```python
from build123d import *

# Parameters (mm, degrees)
EXTRUDE_1_DEPTH               = 3
HOLE_WIZARD_M2_1_AT_2_COUNT   = 2
HOLE_WIZARD_M2_1_AT_2_PITCH   = 21
PATTERN_LINEAR_1_COUNT        = 3
PATTERN_LINEAR_1_PITCH        = 33
PATTERN_LINEAR_2_COUNT        = 3
PATTERN_LINEAR_2_PITCH        = 10.5
PATTERN_LINEAR_3_COUNT        = 2
PATTERN_LINEAR_3_PITCH        = 31.5
HOLE_WIZARD_M2_1_2_AT_2_COUNT = 2
HOLE_WIZARD_M2_1_2_AT_2_PITCH = 16.970562748
SKETCH_8_R                    = 17
CUT_EXTRUDE_1_DEPTH           = 1
SKETCH_9_R                    = 2.025
CUT_EXTRUDE_2_DEPTH           = 75.994999833
PATTERN_CIRCULAR_1_COUNT      = 2
PATTERN_CIRCULAR_1_ANGLE      = 90
FILLET_1_R                    = 4
CHAMFER_1_SIZE                = 1
SKETCH_11_W                   = 95
SKETCH_11_H                   = 18
CUT_EXTRUDE_3_DEPTH           = 76.028327984


with BuildPart() as part:
    # ｽｹｯﾁ1 → ﾎﾞｽ - 押し出し1 (new body)
    with BuildSketch(Plane(origin=(0, 0, 0), x_dir=(1, 0, 0), z_dir=(0, 1, 0))):
        with BuildLine():
            Line((-10.05, 0), (-39, 0))
            Line((-39, 0), (-47.5, 8.5))
            Line((-47.5, 8.5), (-47.5, 58))
            Line((-47.5, 58), (47.5, 58))
            Line((47.5, 58), (47.5, 8.5))
            Line((47.5, 8.5), (39, 0))
            Line((39, 0), (10.05, 0))
            ThreePointArc((10.05, 0), (0, 10.05), (-10.05, 0))
        make_face()
    extrude(amount=EXTRUDE_1_DEPTH)

    # ｽｹｯﾁ3 → Hole Wizard M2 _1 (revolve, cut)
    with BuildSketch(Plane(origin=(-43.5, 3, -54), x_dir=(0, 0, 1), z_dir=(1, 0, 0))):
        Polygon((0, 0), (0, 4.63090365), (1.05, 4), (1.05, 1), (2, 1), (2, 0), align=None)
    hole_wizard_m2_1 = revolve(axis=Axis((-43.5, 9.35, -54), (0, -1, 0)), mode=Mode.SUBTRACT)

    # Hole Wizard M2 _1 at 2: Hole Wizard M2 _1 ×2
    with Locations(*[(i * HOLE_WIZARD_M2_1_AT_2_PITCH, 0, 0) for i in range(1, HOLE_WIZARD_M2_1_AT_2_COUNT)]):
        add(hole_wizard_m2_1, mode=Mode.SUBTRACT)

    # 直線ﾊﾟﾀｰﾝ1: Hole Wizard M2 _1 ×3
    with Locations(*[(i * PATTERN_LINEAR_1_PITCH, 0, 0) for i in range(1, PATTERN_LINEAR_1_COUNT)]):
        add(hole_wizard_m2_1, mode=Mode.SUBTRACT)

    # 直線ﾊﾟﾀｰﾝ1 copy 1 sketch → 直線ﾊﾟﾀｰﾝ1 copy 1 (revolve, cut)
    with BuildSketch(Plane(origin=(10.5, 3, -54), x_dir=(0, 0, 1), z_dir=(1, 0, 0))):
        Polygon((0, 0), (0, 4.63090365), (1.05, 4), (1.05, 1), (2, 1), (2, 0), align=None)
    revolve(axis=Axis((10.5, 9.35, -54), (0, -1, 0)), mode=Mode.SUBTRACT)

    # 直線ﾊﾟﾀｰﾝ1 copy 2 sketch → 直線ﾊﾟﾀｰﾝ1 copy 2 (revolve, cut)
    with BuildSketch(Plane(origin=(43.5, 3, -54), x_dir=(0, 0, 1), z_dir=(1, 0, 0))):
        Polygon((0, 0), (0, 4.63090365), (1.05, 4), (1.05, 1), (2, 1), (2, 0), align=None)
    revolve(axis=Axis((43.5, 9.35, -54), (0, -1, 0)), mode=Mode.SUBTRACT)

    # 直線ﾊﾟﾀｰﾝ2: Hole Wizard M2 _1 ×3
    with Locations(*[(0, 0, i * PATTERN_LINEAR_2_PITCH) for i in range(1, PATTERN_LINEAR_2_COUNT)]):
        add(hole_wizard_m2_1, mode=Mode.SUBTRACT)

    # 直線ﾊﾟﾀｰﾝ2 copy 1 sketch → 直線ﾊﾟﾀｰﾝ2 copy 1 (revolve, cut)
    with BuildSketch(Plane(origin=(-22.5, 3, -43.5), x_dir=(0, 0, 1), z_dir=(1, 0, 0))):
        Polygon((0, 0), (0, 4.63090365), (1.05, 4), (1.05, 1), (2, 1), (2, 0), align=None)
    revolve(axis=Axis((-22.5, 9.35, -43.5), (0, -1, 0)), mode=Mode.SUBTRACT)

    # 直線ﾊﾟﾀｰﾝ2 copy 2 sketch → 直線ﾊﾟﾀｰﾝ2 copy 2 (revolve, cut)
    with BuildSketch(Plane(origin=(-22.5, 3, -33), x_dir=(0, 0, 1), z_dir=(1, 0, 0))):
        Polygon((0, 0), (0, 4.63090365), (1.05, 4), (1.05, 1), (2, 1), (2, 0), align=None)
    revolve(axis=Axis((-22.5, 9.35, -33), (0, -1, 0)), mode=Mode.SUBTRACT)

    # 直線ﾊﾟﾀｰﾝ2 copy 3 sketch → 直線ﾊﾟﾀｰﾝ2 copy 3 (revolve, cut)
    with BuildSketch(Plane(origin=(-10.5, 3, -43.5), x_dir=(0, 0, 1), z_dir=(1, 0, 0))):
        Polygon((0, 0), (0, 4.63090365), (1.05, 4), (1.05, 1), (2, 1), (2, 0), align=None)
    revolve(axis=Axis((-10.5, 9.35, -43.5), (0, -1, 0)), mode=Mode.SUBTRACT)

    # 直線ﾊﾟﾀｰﾝ2 copy 4 sketch → 直線ﾊﾟﾀｰﾝ2 copy 4 (revolve, cut)
    with BuildSketch(Plane(origin=(-10.5, 3, -33), x_dir=(0, 0, 1), z_dir=(1, 0, 0))):
        Polygon((0, 0), (0, 4.63090365), (1.05, 4), (1.05, 1), (2, 1), (2, 0), align=None)
    revolve(axis=Axis((-10.5, 9.35, -33), (0, -1, 0)), mode=Mode.SUBTRACT)

    # 直線ﾊﾟﾀｰﾝ2 copy 5 sketch → 直線ﾊﾟﾀｰﾝ2 copy 5 (revolve, cut)
    with BuildSketch(Plane(origin=(22.5, 3, -43.5), x_dir=(0, 0, 1), z_dir=(1, 0, 0))):
        Polygon((0, 0), (0, 4.63090365), (1.05, 4), (1.05, 1), (2, 1), (2, 0), align=None)
    revolve(axis=Axis((22.5, 9.35, -43.5), (0, -1, 0)), mode=Mode.SUBTRACT)

    # 直線ﾊﾟﾀｰﾝ2 copy 6 sketch → 直線ﾊﾟﾀｰﾝ2 copy 6 (revolve, cut)
    with BuildSketch(Plane(origin=(22.5, 3, -33), x_dir=(0, 0, 1), z_dir=(1, 0, 0))):
        Polygon((0, 0), (0, 4.63090365), (1.05, 4), (1.05, 1), (2, 1), (2, 0), align=None)
    revolve(axis=Axis((22.5, 9.35, -33), (0, -1, 0)), mode=Mode.SUBTRACT)

    # 直線ﾊﾟﾀｰﾝ2 copy 7 sketch → 直線ﾊﾟﾀｰﾝ2 copy 7 (revolve, cut)
    with BuildSketch(Plane(origin=(10.5, 3, -43.5), x_dir=(0, 0, 1), z_dir=(1, 0, 0))):
        Polygon((0, 0), (0, 4.63090365), (1.05, 4), (1.05, 1), (2, 1), (2, 0), align=None)
    revolve(axis=Axis((10.5, 9.35, -43.5), (0, -1, 0)), mode=Mode.SUBTRACT)

    # 直線ﾊﾟﾀｰﾝ2 copy 8 sketch → 直線ﾊﾟﾀｰﾝ2 copy 8 (revolve, cut)
    with BuildSketch(Plane(origin=(10.5, 3, -33), x_dir=(0, 0, 1), z_dir=(1, 0, 0))):
        Polygon((0, 0), (0, 4.63090365), (1.05, 4), (1.05, 1), (2, 1), (2, 0), align=None)
    revolve(axis=Axis((10.5, 9.35, -33), (0, -1, 0)), mode=Mode.SUBTRACT)

    # 直線ﾊﾟﾀｰﾝ2 copy 9 sketch → 直線ﾊﾟﾀｰﾝ2 copy 9 (revolve, cut)
    with BuildSketch(Plane(origin=(43.5, 3, -43.5), x_dir=(0, 0, 1), z_dir=(1, 0, 0))):
        Polygon((0, 0), (0, 4.63090365), (1.05, 4), (1.05, 1), (2, 1), (2, 0), align=None)
    revolve(axis=Axis((43.5, 9.35, -43.5), (0, -1, 0)), mode=Mode.SUBTRACT)

    # 直線ﾊﾟﾀｰﾝ2 copy 10 sketch → 直線ﾊﾟﾀｰﾝ2 copy 10 (revolve, cut)
    with BuildSketch(Plane(origin=(43.5, 3, -33), x_dir=(0, 0, 1), z_dir=(1, 0, 0))):
        Polygon((0, 0), (0, 4.63090365), (1.05, 4), (1.05, 1), (2, 1), (2, 0), align=None)
    revolve(axis=Axis((43.5, 9.35, -33), (0, -1, 0)), mode=Mode.SUBTRACT)

    # 直線ﾊﾟﾀｰﾝ3: Hole Wizard M2 _1 ×2
    with Locations(*[(0, 0, i * PATTERN_LINEAR_3_PITCH) for i in range(1, PATTERN_LINEAR_3_COUNT)]):
        add(hole_wizard_m2_1, mode=Mode.SUBTRACT)

    # 直線ﾊﾟﾀｰﾝ3 copy 1 sketch → 直線ﾊﾟﾀｰﾝ3 copy 1 (revolve, cut)
    with BuildSketch(Plane(origin=(-22.5, 3, -22.5), x_dir=(0, 0, 1), z_dir=(1, 0, 0))):
        Polygon((0, 0), (0, 4.63090365), (1.05, 4), (1.05, 1), (2, 1), (2, 0), align=None)
    revolve(axis=Axis((-22.5, 9.35, -22.5), (0, -1, 0)), mode=Mode.SUBTRACT)

    # ｽｹｯﾁ5 → Hole Wizard M2 _1 2 (revolve, cut)
    with BuildSketch(Plane(origin=(-10.5, 3, -22.5), x_dir=(0, 0, 1), z_dir=(1, 0, 0))):
        Polygon((0, 0), (0, 6.480688495), (0.8, 6), (0.8, 0), align=None)
    hole_wizard_m2_1_2 = revolve(axis=Axis((-10.5, 9.35, -22.5), (0, -1, 0)), mode=Mode.SUBTRACT)

    # Hole Wizard M2 _1 2 at 2: Hole Wizard M2 _1 2 ×2
    with Locations(*[Vector(-0.7071067811865469, 0, 0.7071067811865482) * (i * HOLE_WIZARD_M2_1_2_AT_2_PITCH) for i in range(1, HOLE_WIZARD_M2_1_2_AT_2_COUNT)]):
        add(hole_wizard_m2_1_2, mode=Mode.SUBTRACT)

    # ｽｹｯﾁ7 → M2 なべ頭ねじ用座ぐり穴2 (revolve, cut)
    with BuildSketch(Plane(origin=(-43.5, 3, -12), x_dir=(0, 0, 1), z_dir=(1, 0, 0))):
        Polygon((0, 0), (0, 6.63090365), (1.05, 6), (1.05, 1), (2, 1), (2, 0), align=None)
    hole_wizard_m2_2 = revolve(axis=Axis((-43.5, 9.35, -12), (0, -1, 0)), mode=Mode.SUBTRACT)

    # ﾐﾗｰ1: Hole Wizard M2 _1 2, M2 なべ頭ねじ用座ぐり穴2 across plane
    add(hole_wizard_m2_1_2.mirror(Plane(origin=(0, 0, 0), x_dir=(0, 0, 1), z_dir=(1, 0, 0))), mode=Mode.SUBTRACT)
    add(hole_wizard_m2_2.mirror(Plane(origin=(0, 0, 0), x_dir=(0, 0, 1), z_dir=(1, 0, 0))), mode=Mode.SUBTRACT)

    # ﾐﾗｰ1 copy 1 sketch → ﾐﾗｰ1 copy 1 (revolve, cut)
    with BuildSketch(Plane(origin=(43.5, 3, -22.5), x_dir=(0, 0, 1), z_dir=(-1, 0, 0))):
        Polygon((0, 0), (0, -4.63090365), (1.05, -4), (1.05, -1), (2, -1), (2, 0), align=None)
    revolve(axis=Axis((43.5, 9.35, -22.5), (0, 1, 0)), mode=Mode.SUBTRACT)

    # ﾐﾗｰ1 copy 2 sketch → ﾐﾗｰ1 copy 2 (revolve, cut)
    with BuildSketch(Plane(origin=(22.5, 3, -22.5), x_dir=(0, 0, 1), z_dir=(-1, 0, 0))):
        Polygon((0, 0), (0, -4.63090365), (1.05, -4), (1.05, -1), (2, -1), (2, 0), align=None)
    revolve(axis=Axis((22.5, 9.35, -22.5), (0, 1, 0)), mode=Mode.SUBTRACT)

    # ﾐﾗｰ1 copy 3 sketch → ﾐﾗｰ1 copy 3 (revolve, cut)
    with BuildSketch(Plane(origin=(43.5, 3, -54), x_dir=(0, 0, 1), z_dir=(-1, 0, 0))):
        Polygon((0, 0), (0, -4.63090365), (1.05, -4), (1.05, -1), (2, -1), (2, 0), align=None)
    revolve(axis=Axis((43.5, 9.35, -54), (0, 1, 0)), mode=Mode.SUBTRACT)

    # ﾐﾗｰ1 copy 4 sketch → ﾐﾗｰ1 copy 4 (revolve, cut)
    with BuildSketch(Plane(origin=(22.5, 3, -54), x_dir=(0, 0, 1), z_dir=(-1, 0, 0))):
        Polygon((0, 0), (0, -4.63090365), (1.05, -4), (1.05, -1), (2, -1), (2, 0), align=None)
    revolve(axis=Axis((22.5, 9.35, -54), (0, 1, 0)), mode=Mode.SUBTRACT)

    # ﾐﾗｰ1 copy 5 sketch → ﾐﾗｰ1 copy 5 (revolve, cut)
    with BuildSketch(Plane(origin=(22.5, 3, -10.5), x_dir=(0, 0, 1), z_dir=(-1, 0, 0))):
        Polygon((0, 0), (0, -6.480688495), (0.8, -6), (0.8, 0), align=None)
    revolve(axis=Axis((22.5, 9.35, -10.5), (0, 1, 0)), mode=Mode.SUBTRACT)

    # ｽｹｯﾁ8 → ｶｯﾄ - 押し出し1 (cut)
    with BuildSketch(Plane(origin=(0, 3, 0), x_dir=(1, 0, 0), z_dir=(0, 1, 0))):
        Circle(SKETCH_8_R)
    extrude(amount=-CUT_EXTRUDE_1_DEPTH, mode=Mode.SUBTRACT)

    # ｽｹｯﾁ9 → ｶｯﾄ - 押し出し2 (cut, through all)
    with BuildSketch(Plane(origin=(0, 2, 0), x_dir=(1, 0, 0), z_dir=(0, 1, 0))):
        with Locations(Location((-9.899494937, 9.899494937, 0), (0, 0, 270))):
            Circle(SKETCH_9_R)
    cut_extrude_2 = extrude(amount=-CUT_EXTRUDE_2_DEPTH, mode=Mode.SUBTRACT)

    # 円形ﾊﾟﾀｰﾝ1: ｶｯﾄ - 押し出し2 ×2 about axis
    pattern_circular_1_axis = Axis((0, 3, 0), (0, -1, 0))
    for i in range(1, PATTERN_CIRCULAR_1_COUNT):
        add(cut_extrude_2.rotate(pattern_circular_1_axis, i * PATTERN_CIRCULAR_1_ANGLE / (PATTERN_CIRCULAR_1_COUNT - 1)), mode=Mode.SUBTRACT)

    # ﾌｨﾚｯﾄ1
    fillet_1_edges = [part.edges().sort_by_distance(p)[0] for p in [
        (-47.5, 1.5, -8.5),
        (-47.5, 1.5, -58),
        (47.5, 1.5, -58),
        (47.5, 1.5, -8.5),
        (39, 1.5, 0),
        (-39, 1.5, 0),
    ]]
    fillet(fillet_1_edges, radius=FILLET_1_R)

    # 面取り1
    chamfer_1_edges = [part.edges().sort_by_distance(p)[0] for p in [
        (0, 3, -17),
        (27.171572875, 3, 0),
        (38.87387948, 3, -0.30448187),
        (43.25, 3, -4.25),
        (47.19551813, 3, -8.62612052),
        (47.5, 3, -32.078427125),
        (-27.171572875, 3, 0),
        (46.328427125, 3, -56.828427125),
        (-38.87387948, 3, -0.30448187),
        (0, 3, -58),
        (-43.25, 3, -4.25),
        (-46.328427125, 3, -56.828427125),
        (-47.19551813, 3, -8.62612052),
        (-47.5, 3, -32.078427125),
    ]]
    chamfer(chamfer_1_edges, length=CHAMFER_1_SIZE - 0.0001)  # a hair under: the kernel refuses the full size

    # ｽｹｯﾁ11 → ｶｯﾄ - 押し出し3 (cut, through all)
    with BuildSketch(Plane(origin=(0, 3, 0), x_dir=(1, 0, 0), z_dir=(0, 1, 0))):
        Rectangle(SKETCH_11_W, SKETCH_11_H)
    extrude(amount=-CUT_EXTRUDE_3_DEPTH, mode=Mode.SUBTRACT)


solid = part.part
```
Read the model definition and answer for the solid it produces. Units are mm, in the model's axes. A direction names the side the tool comes from. Round coordinates to 2 decimals unless told otherwise and drop trailing zeros. Answer in a Markdown table with one row per item. Add a question column.
1) Determine the mould class of faces 3 (the face through (-6, 1, -9)), 4 (the face through (10.18, 1.01, -53)), 5 (the face through (11.4, 2, -44.4)), 6 (the face through (-46.359, 1.014, -56.797)) for opening direction X: pulls with the +X half, pulls with the -X half, needs draft (parallel to the pull), parting line crosses it, or undercut.
2) Consider line 1 (Z direction, x = -10.5, y = 1.1); line 2 (Z direction, x = -43, y = 1.15); line 3 (X direction, y = 0.85, z = -12.5). Determine where each line is inside the solid, lowest interval first.
3) Which of the six approach directions +Z, -Z, +X, -X, +Y, -Y give full straight-line access (tool end or side, diameter ignored) to faces 1 (the face through (-47.5, 1, -32)), 2 (the face through (45.274, 2.507, -32.077))?
4) Find section A-A, the plane z = -33. State how many separate pieces and enclosed holes the cut face has, and give its area (3 significant figures).
5) Given P1, Ø3.5, axis at x = 22.5, z = -22.5, coming from the +Y side; P2, Ø1.7, axis at x = -10.5, z = -43.5, coming from the +Y side, each flat-ended and moving along its own axis, determine where each tip first touches the part or whether it passes through.
Findings below:
| question | item | result |
|---|---|---|
| 1 | face 3 | needs draft |
| 1 | face 4 | undercut |
| 1 | face 5 | undercut |
| 1 | face 6 | pulls with the -X half |
| 2 | line 1 | -58 to -55.05, -52.95 to -44.55, -42.45 to -34.05, -31.95 to -23.3, -21.7 to -11.83 |
| 2 | line 2 | -58 to -54.92, -53.08 to -44.42, -42.58 to -33.92, -32.08 to -23.42, -21.58 to -12.92, -11.08 to -9 |
| 2 | line 3 | -47.5 to -44.42, -42.58 to 42.58, 44.42 to 47.5 |
| 3 | face 1 | +Z, -Z, -X, +Y, -Y |
| 3 | face 2 | +Y |
| 4 | separate pieces | 7 |
| 4 | enclosed holes | 0 |
| 4 | area | 235 mm² |
| 5 | P1 | y = 2 |
| 5 | P2 | through |
